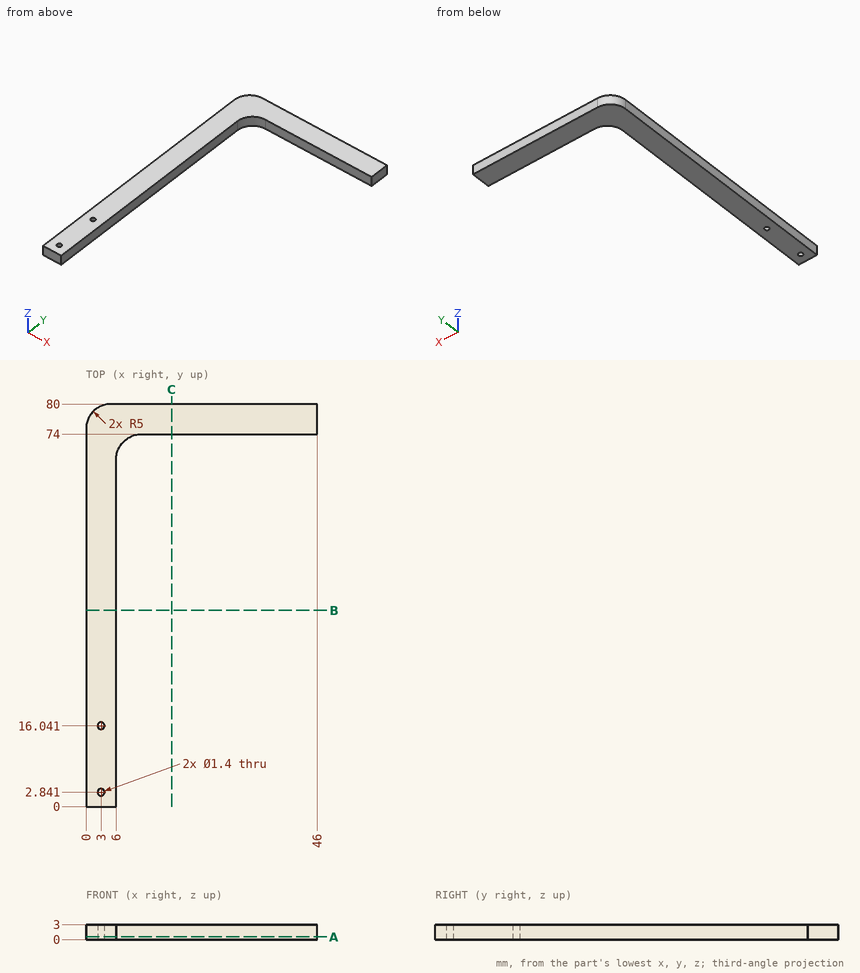
The drawing under review shows one solid part. Ordinate dimensions are in mm from its lowest x, y, z. Give positions to 0.01 mm unless a question says otherwise; leave off trailing zeros. Loops run counter-clockwise (first coordinate to the right, second up) from the corner with the lowest first, then second, coordinate; pieces in that order, holes last. Notation, with made-up numbers: M 89.25,-10.5 L 124.25,-10.5 A27 cw 124.25,12.5 Z; hole C -23.75,-9.75 d11. An arc over 180 degrees is marked long. One line per item, written item: value. Start each with the question number.
Q1. Clearance check with a flat-ended pin moving along its axis: pin 1 Ø1.5 at (y, z) = (42, 2) entering from +X. State where the tip first meets the part, or that it passes through.
Q2. Add section C-C (x = 17). Give the boundary of the cut face in (y, z), and give its area (3 significant figures).
Q3. Add section A-A (z = 0.55). Give the boundary of the cut face in (x, y).
Q4. Add section B-B (y = 39). Give the boundary of the cut face in (x, z).
Q5. For L1, parallel to Y at x = 3, z = 0.8; L2, parallel to Y at x = 43, z = 1.45; L3, parallel to X at y = 44.5, z = 1.05, list the stretches that pass through material, from the lowest coordinate up.
Reply:
1. pin 1: x = 6
2. outline: M 74,0 L 80,0 L 80,3 L 74,3 Z
2. area: 18.0 mm²
3. outline: M 0,0 L 6,0 L 6,69 A5 cw 11,74 L 46,74 L 46,80 L 5,80 A5 ccw 0,75 Z; hole C 3,2.84 d1.4; hole C 3,16.04 d1.4
4. outline: M 0,0 L 6,0 L 6,3 L 0,3 Z
5. L1: 0 to 2.14, 3.54 to 15.34, 16.74 to 79.58
5. L2: 74 to 80
5. L3: 0 to 6
